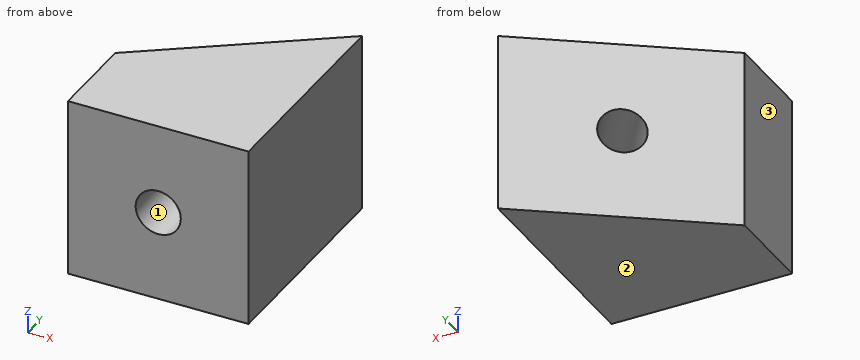
Autodesk Inventor part; units mm, degrees
ref_plane "YZ Plane" through (0, 0, 0) normal (1, 0, 0) x (0, 1, 0)
ref_plane "XZ Plane" through (0, 0, 0) normal (0, 1, 0) x (-1, 0, 0)
ref_plane "XY Plane" through (0, 0, 0) normal (0, 0, 1) x (1, 0, 0)
sketch "Sketch1" plane through (0, 0, 0) normal (0, 0, 1) x (1, 0, 0)
  line L0 (-16.2275, -3.6228) -> (9.1725, 14.1625)
  line L1 (9.1725, 14.1625) -> (9.1725, -16.3228)
  line L2 (9.1725, -16.3228) -> (-16.2275, -16.3228)
  line L3 (-16.2275, -16.3228) -> (-16.2275, -3.6228)
  dimension "d6" = 35
  dimension "d7" = 12.7
  dimension "d8" = 25.4
extrude "Extrusion1" add sketch "Sketch1" along normal blind 25.4
sketch "Sketch2" plane through (9.1725, 14.1625, 25.4) normal (-0.5736, 0.8192, 0) x (0.8192, 0.5736, 0)
  circle A0 centre (-15.6369, 12.7) radius 3.175
  point P0 (-15.6369, 25.4)
  dimension "d11" = 6.35
extrude "Extrusion2" cut sketch "Sketch2" against normal blind 12.7
sketch "Sketch3" plane through (-16.2275, -16.3228, 0) normal (0, -1, 0) x (1, 0, 0)
  circle A0 centre (12.7, 12.7) radius 3.175
  point P0 (16.2275, 0)
  dimension "d14" = 6.35
extrude "Extrusion3" cut sketch "Sketch3" against normal blind 10.16
properties part number "hack 35 degree mounting points"
Can you work these out from the model? Positions are in its coordinate system, mm. Face numbers are marked on the shaded views. Coordinates: 2 decimals unless noted, no trailing zeros. Loops run counter-clockwise (first coordinate to the right, second up) from the corner with the lowest first, then second, coordinate; pieces in that order, holes last.
1) Imagine slicing it at C-C on z = 3.5. List the corners of the cut face in (x, y) for me, plus the area to 3 significant figures.
2) Imagine slicing it at A-A on z = 11.25. List the corners of the cut face in (x, y) for me, plus the area to 3 significant figures.
3) Thinking about a two-plate mould opening in X: for the marked faces 1, 2 and 3, which applies, pulls with the +X half, pulls with the -X half, needs draft (parallel to the pull), parting line crosses it, or undercut?
4) For pin 1 (10 mm diameter, centred on y = 2.5, z = 11.5, fed in from -X); pin 2 (5 mm diameter, centred on x = -7.5, z = 21, fed in from +Y); pin 3 (5 mm diameter, centred on x = -3.53, z = 12.7, fed in from -Y), each with a flat end and sliding along its axis, tell me the tip position at first contact or that it passes through.
5) Imagine slicing it at B-B on x = -12.5. List the corners of the cut face in (y, z) for me, plus the area to 3 significant figures.
6) I need wall thicknesses on probe 1 along X at (y, z) = (0, 11); probe 2 along X at (y, z) = (-8, 12.75); probe 3 along Z at (x, y) = (-4, -7.5). Which ranges of each line are inside material? Lowest first, please.
Completed:
1. outline: (-16.23, -16.32) - (9.17, -16.32) - (9.17, 14.16) - (-16.23, -3.62) - close
1. area: 548 mm2
2. outline: (-16.23, -16.32) - (-6.35, -16.32) - (-6.35, -6.16) - (-0.7, -6.16) - (-0.7, -16.32) - (9.17, -16.32) - (9.17, 14.16) - (-1.32, 6.81) - (5.96, -3.59) - (1.34, -6.83) - (-5.95, 3.57) - (-16.23, -3.62) - close
2. area: 419 mm2
3. face 1: undercut
3. face 2: needs draft
3. face 3: pulls with the -X half
4. pin 1: stops at x = -14.62
4. pin 2: stops at y = 4.24
4. pin 3: stops at y = -6.16
5. outline: (-16.32, 0) - (-1.01, 0) - (-1.01, 25.4) - (-16.32, 25.4) - close
5. area: 389 mm2
6. probe 1: x = -11.05 to -3.27, 3.27 to 9.17
6. probe 2: x = -16.23 to -6.7, -0.35 to 9.17
6. probe 3: z = 0 to 9.56, 15.84 to 25.4
